CAD build for the part. Positions are in the model's coordinates, mm. Face numbers are marked on the shaded views. Coordinates: 2 decimals unless noted, no trailing zeros. Loops run counter-clockwise (first coordinate to the right, second up) from the corner with the lowest first, then second, coordinate; pieces in that order, holes last. Notation, with made-up numbers: M 75.25,9.25 L 123.25,9.25 A19 cw 123.25,46.25 Z; hole C -27.5,-39.75 d10. An arc over 180 degrees is marked long. Answer as a JSON object with one key per item and string values. Group by question number.
Autodesk Inventor part; units mm, degrees
ref_plane "YZ Plane" through (0, 0, 0) normal (1, 0, 0) x (0, 1, 0)
ref_plane "XZ Plane" through (0, 0, 0) normal (0, 1, 0) x (-1, 0, 0)
ref_plane "XY Plane" through (0, 0, 0) normal (0, 0, 1) x (1, 0, 0)
sketch "Sketch1" plane through (0, 0, 0) normal (0, 1, 0) x (-1, 0, 0)
  line L0 (-20, 20) -> (20, 20)
  line L1 (20, 20) -> (20, -20)
  line L2 (20, -20) -> (-20, -20)
  line L3 (-20, -20) -> (-20, 20)
  line L4 (-20, 20) -> (20, -20) construction
  line L5 (20, 20) -> (-20, -20) construction
  circle A0 centre (0, 0) radius 4
  circle A1 centre (0, 8.5) radius 1.75
  circle A2 centre (0, -8.5) radius 1.75
  point P0 (0, 0)
  point P1 (0, 0)
  dimension "d0" = 40
  dimension "d1" = 40
  dimension "d2" = 8
  dimension "d3" = 3.5
  dimension "d4" = 3.5
  dimension "d5" = 8.5
  dimension "d6" = 8.5
extrude "Extrusion1" add sketch "Sketch1" along normal blind 3
chamfer "Chamfer1" distance 2 angle 45 2 edges at (1.75, 3, -8.5) (1.75, 3, 8.5)
sketch "Sketch3" plane through (0, 3, 0) normal (0, 1, 0) x (1, 0, 0)
  circle A0 centre (-15, -15) radius 1.75
  circle A1 centre (-15, 15) radius 1.75
  circle A2 centre (15, 15) radius 1.75
  circle A3 centre (15, -15) radius 1.75
  point P0 (0, 0)
  dimension "d13" = 3.5
  dimension "d14" = 15
  dimension "d15" = 15
  dimension "d16" = 15
  dimension "d17" = 15
extrude "Extrusion2" cut sketch "Sketch3" against normal through all
sketch "Sketch4" plane through (0, 3, 0) normal (0, 1, 0) x (1, 0, 0)
  circle A0 centre (0, 0) radius 11.5
  dimension "d20" = 23
extrude "Extrusion3" cut sketch "Sketch4" against normal blind 10
sketch "Sketch5" plane through (0, 3, 0) normal (0, 1, 0) x (1, 0, 0)
  circle A0 centre (0, 0) radius 11.5
  circle A1 centre (0, 0) radius 12.5
  arc A2 (2.6001, -11.2022) -> (2.6001, 11.2022) centre (0, 0) ccw
  dimension "d23" = 1
extrude "Extrusion4" add sketch "Sketch5" along normal mid plane 2
fillet "Fillet2" radius 8 2 edges at (-20, 1.5, 20) (20, 1.5, 20)
fillet "Fillet3" radius 1 2 edges at (20, 1.5, -20) (-20, 1.5, -20)
properties part number "soportemotor"
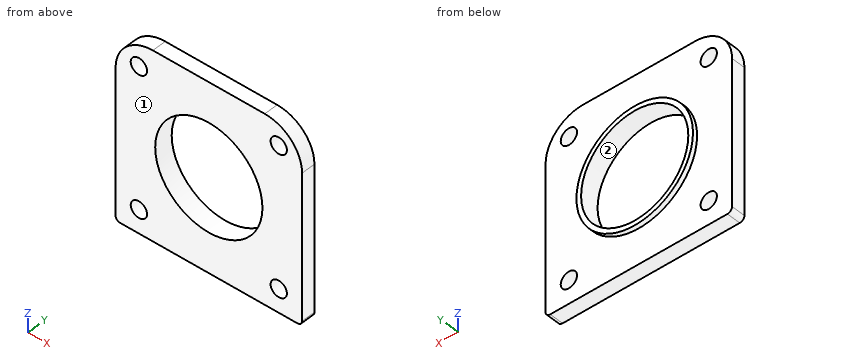
Item 1: Slice it at B-B, the plane x = 0. Write the cut outline in (y, z), then the cut area to 3 significant figures.
Item 2: Slice it at C-C, the plane z = -15. Write the cut outline in (x, y).
Item 3: Slice it at A-A, the plane z = 0. Write the cut outline in (x, y), then the cut area to 3 significant figures.
Item 4: Pin check, flat tip, straight feed: pin 1 (4 mm diameter, centred on x = -15, z = 15, fed in from +Y). Stop position of the tip, or through.
Item 5: Drill centre lines: L1, parallel to X at y = 1.55, z = -15; L2, parallel to X at y = 2.5, z = 14.5; L3, parallel to Z at x = -15, y = 1.2. Where is each one in solid material? Low to high. Write a range as from..to.
Item 6: Pull direction Z, two halves, no side cores. Call the marked faces 1 and 2: released by +Z, released by -Z, zero draft, split by the parting line, or undercut.
Item 7: Slice it at D-D, the plane y = 0.7. Write the cut outline in (x, z), then the cut area to 3 significant figures.
Computed:
{
 "1": {"outline": "M 0,-20 L 3,-20 L 3,-12.5 L 4,-12.5 L 4,-11.5 L 0,-11.5 Z; M 0,11.5 L 4,11.5 L 4,12.5 L 3,12.5 L 3,20 L 0,20 Z", "area": "53.0 mm2"},
 "2": {"outline": "M -20,0 L -16.75,0 L -16.75,3 L -20,3 Z; M -13.25,0 L 13.25,0 L 13.25,3 L -13.25,3 Z; M 16.75,0 L 20,0 L 20,3 L 16.75,3 Z"},
 "3": {"outline": "M -20,0 L -11.5,0 L -11.5,4 L -12.5,4 L -12.5,3 L -20,3 Z; M 11.5,0 L 20,0 L 20,3 L 12.5,3 L 12.5,4 L 11.5,4 Z", "area": "53.0 mm2"},
 "4": {"pin 1": "y = 3"},
 "5": {"L1": "-20..-16.75, -13.25..13.25, 16.75..20", "L2": "-19.6..-16.68, -13.32..13.32, 16.68..19.6", "L3": "-20..-16.75, -13.25..13.25, 16.75..19.42"},
 "6": {"face 1": "zero draft", "face 2": "undercut"},
 "7": {"outline": "M -20,-19 A1 ccw -19,-20 L 19,-20 A1 ccw 20,-19 L 20,12 A8 ccw 12,20 L -12,20 A8 ccw -20,12 Z; hole C -15,-15 d3.5; hole C -15,15 d3.5; hole C 0,0 d23; hole C 15,-15 d3.5; hole C 15,15 d3.5", "area": "1,120 mm2"}
}
